```python
from build123d import *

# Parameters (mm, degrees)
SM_BASE_FLANGE_1_DEPTH   = 1963
CUT_EXTRUDE_1_DEPTH      = 2056.095688695
CUT_EXTRUDE_1_DEPTH_BACK = 2056.095688695


# Sheet-metal steps are written as plain solids
with BuildPart() as part:
    # Sketch 1 → Базовая кромка1 (new body)
    with BuildSketch(Plane.XY.offset(978.154266119)):
        with BuildLine():
            ThreePointArc((-78.935450432, 43.826476967), (295.859427587, 605.918755478), (670.654305605, 43.826476967))
            Line((670.654305605, 43.826476967), (671.577445699, 43.442013227))
            ThreePointArc((671.577445699, 43.442013227), (295.859427587, 606.918755478), (-79.858590526, 43.442013227))
            Line((-79.858590526, 43.442013227), (-78.935450432, 43.826476967))
        make_face()
    extrude(amount=-SM_BASE_FLANGE_1_DEPTH)

    # Эскиз6 → Вырез-Вытянуть1 (cut, two sides: drawn at the far end of the back side and taken through both)
    with BuildSketch(Plane(origin=(295.859427587, 199.918755478, 988), x_dir=(0, 0, -1), z_dir=(1, 0, 0)).offset(-CUT_EXTRUDE_1_DEPTH_BACK)):
        Polygon((529.845733881, 406.969134819), (529.845733881, -18.075276179), (699.845733881, -18.030865181), (1434.845733881, 326.969134819), (1434.845733881, 406.969134819), (1434.845733881, 592.56230864), (529.845733881, 592.56230864), align=None)
    extrude(amount=CUT_EXTRUDE_1_DEPTH + CUT_EXTRUDE_1_DEPTH_BACK, mode=Mode.SUBTRACT)


solid = part.part
```
For this review, take the finished solid that the model builds, in its own axes (mm). Give positions to 0.01 mm unless a question says otherwise; leave off trailing zeros. Order: outer loops, then holes, each group sorted by start corner. A loop starts at its lowest first (then second) coordinate and runs counter-clockwise, first axis right, second up.
1) Wall thickness on line 1 (X direction, y = 189.5, z = -495); line 2 (X direction, y = 133, z = 264); line 3 (Y direction, x = 523.5, z = 603): over which ranges is each line inside the solid? List them lowest first.
2) Take a section at D-D (y = 307.5). Give the boundary of the cut face in (x, z).
3) The part is to be moulded in two halves that separate along Y. For faces 1 (the face through (-99.17, 293.66, 10.4)), 2 (the face through (691.862, 293.893, 10.395)), say which applies: released by +Y, released by -Y, zero draft, split by the parting line, or undercut.
4) Take a section at A-A (z = -236.5). Give the boundary of the cut face in (x, y), then the cut area to 3 significant figures.
5) Take a section at C-C (x = 567). Give the boundary of the cut face in (y, z).
6) Insertion check: pin 1 (1 mm diameter, centred on x = 183, z = 637, fed in from -Y); pin 2 (4 mm diameter, centred on x = 43.5, z = -727.5, fed in from +Y); pin 3 (3 mm diameter, centred on y = 312, z = -389, fed in from -X). Each pin has a flat end and moves straight along its axis. Give the tip position at first contact, or say it passes through.
Derived:
1. line 1: x = -111.01 to -110.01, 701.73 to 702.73
1. line 2: x = -105.6 to -104.59, 696.31 to 697.32
1. line 3: y = 536.1 to 537.3
2. outline: (-96.66, -984.85) - (-95.63, -984.85) - (-95.63, 20.55) - (-96.66, 20.55) - close; (-96.66, 458.15) - (-95.63, 458.15) - (-95.63, 978.15) - (-96.66, 978.15) - close; (687.35, -984.85) - (688.38, -984.85) - (688.38, 20.55) - (687.35, 20.55) - close; (687.35, 458.15) - (688.38, 458.15) - (688.38, 978.15) - (687.35, 978.15) - close
3. face 1: undercut
3. face 2: split by the parting line
4. outline: (-79.86, 43.44) - (-78.94, 43.83) arc R406 cw to (-39.92, 428.15) - (-41.12, 428.15) arc R407 ccw to start; (631.63, 428.15) arc R406 cw to (670.65, 43.83) - (671.58, 43.44) arc R407 ccw to (632.84, 428.15) - close
4. area: 806 mm2
5. outline: (502.11, -984.85) - (503.45, -984.85) - (503.45, -396.91) - (502.11, -394.06) - close; (502.11, 458.15) - (503.45, 458.15) - (503.45, 978.15) - (502.11, 978.15) - close
6. pin 1: stops at y = 589.77
6. pin 2: stops at y = 520.81
6. pin 3: stops at x = -95.83
